```python
from build123d import *

# Parameters (mm, degrees)
BOSS_EXTRUDE1_DEPTH = 50
FILLET1_R           = 1
FILLET2_R           = 3
SKETCH2_R           = 2
CUT_EXTRUDE1_DEPTH  = 10
SKETCH4_R           = 11.5
CUT_EXTRUDE3_DEPTH  = 17
SKETCH5_R           = 4.5
CUT_EXTRUDE4_DEPTH  = 3


with BuildPart() as part:
    # Sketch1 → Boss-Extrude1 (new body)
    with BuildSketch(Plane.XY):
        Polygon((-32, -50), (-32, 52), (32, 52), (32, -50), (30, -50), (30, 50), (-30, 50), (-30, -50), align=None)
    extrude(amount=BOSS_EXTRUDE1_DEPTH)

    # Fillet1
    fillet1_edges = [part.edges().sort_by_distance(p)[0] for p in [
        (30, 50, 25),
        (-30, 50, 25),
    ]]
    fillet(fillet1_edges, radius=FILLET1_R)

    # Fillet2
    fillet2_edges = [part.edges().sort_by_distance(p)[0] for p in [
        (-32, 52, 25),
        (32, 52, 25),
    ]]
    fillet(fillet2_edges, radius=FILLET2_R)

    # Sketch2 → Cut-Extrude1 (cut)
    with BuildSketch(Plane(origin=(0, 52, 0), x_dir=(1, 0, 0), z_dir=(0, 1, 0))):
        with Locations(Location((0, -14, 0), (0, 0, 270))):
            Circle(SKETCH2_R)
        with Locations(Location((11, -25, 0), (0, 0, 270))):
            Circle(SKETCH2_R)
        with Locations(Location((0, -36, 0), (0, 0, 270))):
            Circle(SKETCH2_R)
        with Locations(Location((-11, -25, 0), (0, 0, 270))):
            Circle(SKETCH2_R)
    extrude(amount=-CUT_EXTRUDE1_DEPTH, mode=Mode.SUBTRACT)

    # Sketch4 → Cut-Extrude3 (cut)
    with BuildSketch(Plane(origin=(32, 0, 0), x_dir=(0, 0, -1), z_dir=(1, 0, 0))):
        with Locations((-25, -28)):
            Circle(SKETCH4_R)
    extrude(amount=-CUT_EXTRUDE3_DEPTH, mode=Mode.SUBTRACT)

    # Sketch5 → Cut-Extrude4 (cut)
    with BuildSketch(Plane(origin=(-30, 0, 0), x_dir=(0, 0, -1), z_dir=(1, 0, 0))):
        with Locations((-25, -28)):
            Circle(SKETCH5_R)
    extrude(amount=-CUT_EXTRUDE4_DEPTH, mode=Mode.SUBTRACT)


solid = part.part
```
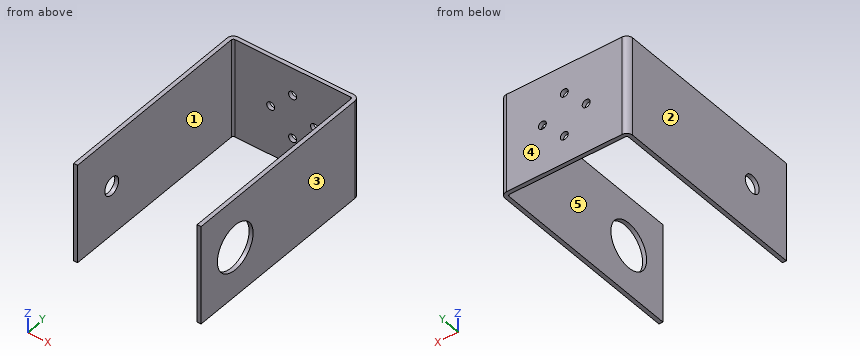
Can you work these out from the model? Positions are in its coordinate system, mm. Face numbers are marked on the shaded views. A direction names the side the tool comes from. Give positions to 0.01 mm unless a question says otherwise; leave off trailing zeros. Loops run counter-clockwise (first coordinate to the right, second up) from the corner with the lowest first, then second, coordinate; pieces in that order, holes last. Notation, with made-up numbers: M -3.75,52 L 50.25,52 A24 ccw 50.25,85 Z; hole C 10.5,-26.5 d11. An arc over 180 degrees is marked long. Use one line per item in the form item = value. Start each with the question number.
(1) I'm going to push flat-ended pins straight in: P1, Ø8, axis at x = -21.5, z = 32, coming from the -Y side; P2, Ø14, axis at y = -28, z = 25, coming from the +X side. Where does each tip first touch, or does it pass through?
(2) On a 3-axis mill with a long thin cutter (end or side, diameter ignored), from which of +Z, -Z, +X, -X, +Y, -Y can I reach the whole of each face in a straight line? I mean the marked faces 1 and 2. Say none if no direction works.
(3) I want a section at D-D, the plane x = 0. Write out the boundary of the cut face in (y, z), and give its area (3 significant figures).
(4) I want a section at A-A, the plane x = -11. Write out the boundary of the cut face in (y, z).
(5) Thinking about a two-plate mould opening in X: for the marked faces 3, 4 and 5, which applies, released by +X, released by -X, zero draft, split by the parting line, or undercut?
(6) Please list where these lines run through material, in increasing order: line 1 (X direction, y = -17, z = 6); line 2 (X direction, y = 51.1, z = 25); line 3 (X direction, y = 51.4, z = 25).
(7) I want a section at C-C, the plane z = 25. Write out the boundary of the cut face in (x, y), and give its area (3 significant figures).
(8) I want a section at B-B, the plane y = 16.5. Write out the boundary of the cut face in (x, z), and give its area (3 significant figures).
Worked out:
q1.P1 = 50
q1.P2 = -30
q2.face_1 = +Z, -Z, -Y
q2.face_2 = +Z, -Z, -X, +Y, -Y
q3.outline = M 50,0 L 52,0 L 52,12 L 50,12 Z; M 50,16 L 52,16 L 52,34 L 50,34 Z; M 50,38 L 52,38 L 52,50 L 50,50 Z
q3.area = 84.0 mm²
q4.outline = M 50,0 L 52,0 L 52,23 L 50,23 Z; M 50,27 L 52,27 L 52,50 L 50,50 Z
q5.face_3 = released by +X
q5.face_4 = zero draft
q5.face_5 = undercut
q6.line_1 = -32 to -30, 30 to 32
q6.line_2 = -31.14 to -13, -9 to 9, 13 to 31.14
q6.line_3 = -30.8 to -13, -9 to 9, 13 to 30.8
q7.outline = M -32,-50 L -30,-50 L -30,-32.5 L -32,-32.5 Z; M -32,-23.5 L -30,-23.5 L -30,49 A1 cw -29,50 L -13,50 L -13,52 L -29,52 A3 ccw -32,49 Z; M -9,50 L 9,50 L 9,52 L -9,52 Z; M 13,50 L 29,50 A1 cw 30,49 L 30,-16.5 L 32,-16.5 L 32,49 A3 ccw 29,52 L 13,52 Z; M 30,-50 L 32,-50 L 32,-39.5 L 30,-39.5 Z
q7.area = 445 mm²
q8.outline = M -32,0 L -30,0 L -30,50 L -32,50 Z; M 30,0 L 32,0 L 32,50 L 30,50 Z
q8.area = 200 mm²
